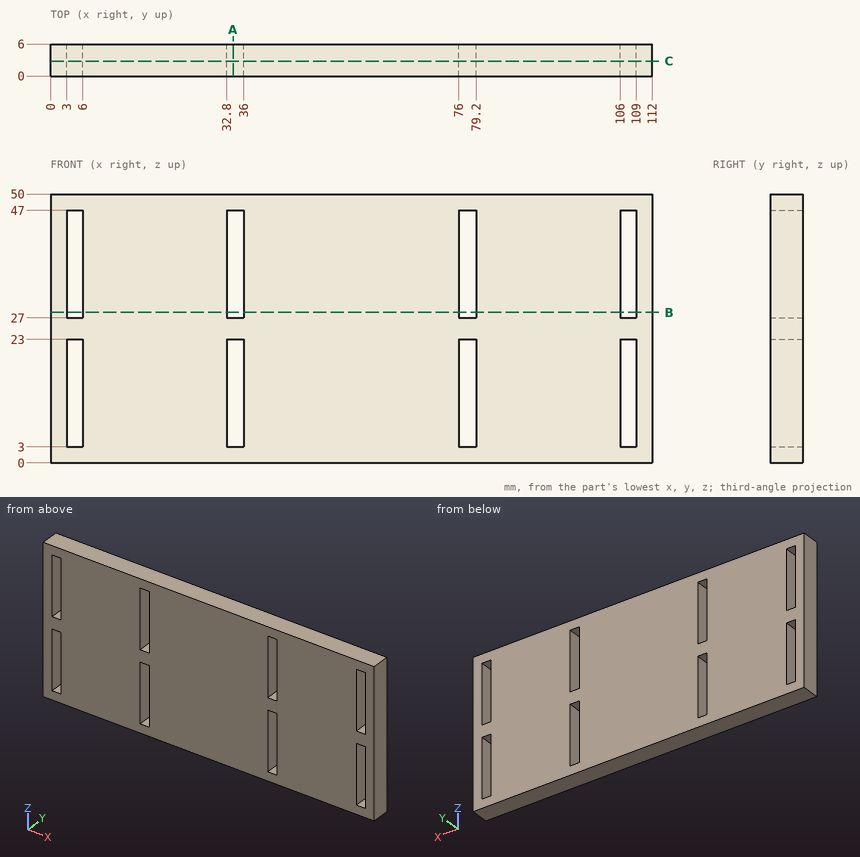
Part print with two shaded views. Sizes in mm from the minimum x, y, z corner. Round coordinates to 2 decimals unless told otherwise and drop trailing zeros. Loops run counter-clockwise (first coordinate to the right, second up) from the corner with the lowest first, then second, coordinate; pieces in that order, holes last.
Item 1: Drill centre lines: line 1 along X through (y, z) = (5.15, 11); line 2 along Z through (x, y) = (78, 1.65). Where is each one in solid material? Low to high.
Item 2: Saw through at B-B (z = 28). List the corners of the cut face in (x, y).
Item 3: Saw through at A-A (x = 34). List the corners of the cut face in (y, z), then the cut area to 3 significant figures.
Item 4: Saw through at C-C (y = 2.8). State how many separate pieces and enclosed holes the cut face has, then the cut area to 3 significant figures.
Worked answers:
1. line 1: x = 0 to 3, 6 to 32.8, 36 to 76, 79.2 to 106, 109 to 112
1. line 2: z = 0 to 3, 23 to 27, 47 to 50
2. outline: (0, 0) - (3, 0) - (3, 6) - (0, 6) - close; (6, 0) - (32.8, 0) - (32.8, 6) - (6, 6) - close; (36, 0) - (76, 0) - (76, 6) - (36, 6) - close; (79.2, 0) - (106, 0) - (106, 6) - (79.2, 6) - close; (109, 0) - (112, 0) - (112, 6) - (109, 6) - close
3. outline: (0, 0) - (6, 0) - (6, 3) - (0, 3) - close; (0, 23) - (6, 23) - (6, 27) - (0, 27) - close; (0, 47) - (6, 47) - (6, 50) - (0, 50) - close
3. area: 60.0 mm2
4. separate pieces: 1
4. enclosed holes: 8
4. area: 5,100 mm2
